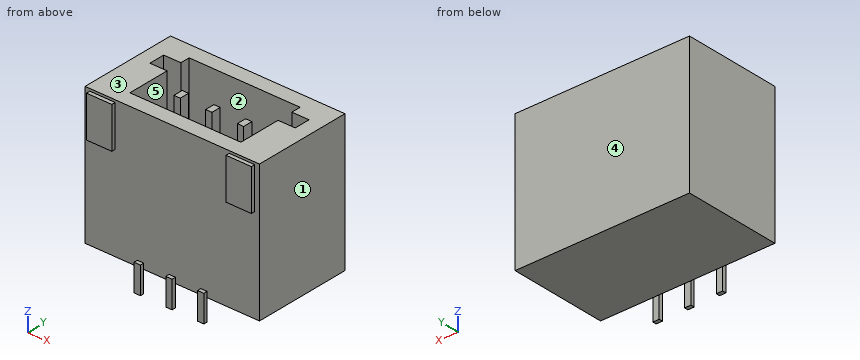
```python
from build123d import *

# Parameters (mm, degrees)
SKETCH_1_W          = 4.35
SKETCH_1_H          = 3.1
EXTRUDE_1_DEPTH     = 5.5
CUT_EXTRUDE_1_DEPTH = 3.7
SKETCH_4_W          = 0.2
SKETCH_4_H          = 0.3
EXTRUDE_2_DEPTH     = 3.5
SKETCH_5_W          = 0.2
SKETCH_5_H          = 0.85
SKETCH_5_W_2        = 0.8
SKETCH_5_H_2        = 1.3
EXTRUDE_3_DEPTH     = 0.12


with BuildPart() as part:
    # 草图1 → 凸台-拉伸1 (new body)
    with BuildSketch(Plane(origin=(0, 0, 0), x_dir=(0, 0, -1), z_dir=(1, 0, 0))):
        with Locations((2.175, 1.55)):
            Rectangle(SKETCH_1_W, SKETCH_1_H)
    extrude(amount=EXTRUDE_1_DEPTH)

    # 草图2 → 切除-拉伸1 (cut)
    with BuildSketch(Plane.XY):
        Polygon((1, 0.475), (4.5, 0.475), (4.5, 1.825), (5.041281958, 1.825), (5.041281958, 2.325), (4.5, 2.325), (4.5, 2.625), (1, 2.625), (1, 2.325), (0.458718042, 2.325), (0.458718042, 1.825), (1, 1.825), align=None)
    extrude(amount=-CUT_EXTRUDE_1_DEPTH, mode=Mode.SUBTRACT)

    # 草图4 → 凸台-拉伸2 (add)
    with BuildSketch(Plane.XY.offset(-3.7)):
        with Locations((2.75, 1.475)):
            Rectangle(SKETCH_4_W, SKETCH_4_H)
        with Locations((1.75, 1.475)):
            Rectangle(SKETCH_4_W, SKETCH_4_H)
        with Locations((3.75, 1.475)):
            Rectangle(SKETCH_4_W, SKETCH_4_H)
    extrude(amount=EXTRUDE_2_DEPTH)

    # 草图5 → 凸台-拉伸3 (add)
    with BuildSketch(Plane.XZ):
        with Locations((2.75, -4.6)):
            Rectangle(SKETCH_5_W, SKETCH_5_H)
        with Locations((0.55, -0.725)):
            Rectangle(SKETCH_5_W_2, SKETCH_5_H_2)
        with Locations((1.75, -4.6)):
            Rectangle(SKETCH_5_W, SKETCH_5_H)
        with Locations((3.75, -4.6)):
            Rectangle(SKETCH_5_W, SKETCH_5_H)
        with Locations((4.95, -0.725)):
            Rectangle(SKETCH_5_W_2, SKETCH_5_H_2)
    extrude(amount=EXTRUDE_3_DEPTH)


solid = part.part
```
Can you work these out from the model? Positions are in its coordinate system, mm. Face numbers are marked on the shaded views. A direction names the side the tool comes from. Round coordinates to 2 decimals unless told otherwise and drop trailing zeros. Loops run counter-clockwise (first coordinate to the right, second up) from the corner with the lowest first, then second, coordinate; pieces in that order, holes last. Notation, with made-up numbers: M -5,1 L 10,1 A11 ccw 10,6 Z; hole C 30,81.5 d9. An arc over 180 degrees is marked long. Answer as a JSON object with one key per item and string values. Group by question number.
Q1. On a 3-axis mill with a long thin cutter (end or side, diameter ignored), from which of +Z, -Z, +X, -X, +Y, -Y can I reach the whole of each face in a straight line? I mean the marked faces 1 and 2. Say none if no direction works.
Q2. Imagine slicing it at D-D, the plane x = 1.15. Please give me the cut outline in (y, z) (3 decimals), then the cut area to 3 significant figures.
Q3. We'd pull the mould along Y, two halves only. Please class the marked faces 3, 4 and 5: +Y half, -Y half, draft (parallel to the pull), parting line (faces both ways), or undercut.
Q4. Imagine slicing it at B-B, the plane x = 4.7. Please give me the cut outline in (y, z) (3 decimals).
Q5. Imagine slicing it at A-A, the plane z = -2.75. Please give me the cut outline in (x, y) (3 decimals).
Q6. Imagine slicing it at C-C, the plane y = 2.15. Please give me the cut outline in (x, z), then the cut area to 3 significant figures.
Q7. Please list where these lines run through material, in increasing order: L1, parallel to Y at x = 2.8, z = -0.5 (3 decimals); L2, parallel to X at y = 2.5, z = -2.85; L3, parallel to Y at x = 2.95, z = -2.95 (3 decimals).
Findings:
{
 "1": {"face 1": "+Z, -Z, +X, +Y, -Y", "face 2": "+Z"},
 "2": {"outline": "M 0,-4.35 L 3.1,-4.35 L 3.1,0 L 2.625,0 L 2.625,-3.7 L 0.475,-3.7 L 0.475,0 L 0,0 Z", "area": "5.53 mm2"},
 "3": {"face 3": "draft", "face 4": "+Y half", "face 5": "undercut"},
 "4": {"outline": "M -0.12,-1.375 L 0,-1.375 L 0,-4.35 L 3.1,-4.35 L 3.1,0 L 2.325,0 L 2.325,-3.7 L 1.825,-3.7 L 1.825,0 L 0,0 L 0,-0.075 L -0.12,-0.075 Z"},
 "5": {"outline": "M 0,0 L 5.5,0 L 5.5,3.1 L 0,3.1 Z; M 1.65,1.325 L 1.85,1.325 L 1.85,1.625 L 1.65,1.625 Z; M 2.65,1.325 L 2.85,1.325 L 2.85,1.625 L 2.65,1.625 Z; M 3.65,1.325 L 3.85,1.325 L 3.85,1.625 L 3.65,1.625 Z; hole M 0.459,1.825 L 1,1.825 L 1,0.475 L 4.5,0.475 L 4.5,1.825 L 5.041,1.825 L 5.041,2.325 L 4.5,2.325 L 4.5,2.625 L 1,2.625 L 1,2.325 L 0.459,2.325 Z"},
 "6": {"outline": "M 0,-4.35 L 5.5,-4.35 L 5.5,0 L 5.04,0 L 5.04,-3.7 L 0.46,-3.7 L 0.46,0 L 0,0 Z", "area": "6.97 mm2"},
 "7": {"L1": "y = 0 to 0.475, 1.325 to 1.625, 2.625 to 3.1", "L2": "x = 0 to 1, 4.5 to 5.5", "L3": "y = 0 to 0.475, 2.625 to 3.1"}
}
